Autodesk Inventor part; units mm, degrees
ref_plane "YZ Plane" through (0, 0, 0) normal (1, 0, 0) x (0, 1, 0)
ref_plane "XZ Plane" through (0, 0, 0) normal (0, 1, 0) x (-1, 0, 0)
ref_plane "XY Plane" through (0, 0, 0) normal (0, 0, 1) x (1, 0, 0)
sketch "Sketch3" plane through (0, 0, 0) normal (0, 1, 0) x (-1, 0, 0)
  line L0 (0, 0) -> (35, 0)
  line L1 (35, 0) -> (35, -45)
  line L2 (35, -45) -> (0, -45)
  line L3 (0, -45) -> (0, 0)
  circle A0 centre (25, -10.5) radius 8.5
  circle A1 centre (25, -34.5) radius 8.5
  line L4 (35, 0) -> (38, 0)
  line L5 (38, 0) -> (38, -45)
  line L6 (38, -45) -> (38, -48)
  line L7 (38, -48) -> (0, -48)
  line L8 (0, -48) -> (-3, -48)
  line L9 (-3, -48) -> (-3, 0)
  line L10 (-3, 0) -> (-3, 3)
  line L11 (-3, 3) -> (38, 3)
  line L12 (38, 3) -> (38, 0)
  dimension "d26" = 45
  dimension "d27" = 35
  dimension "d31" = 17
  dimension "d32" = 17
  dimension "d33" = 3
  dimension "d34" = 3
  dimension "d35" = 3
  dimension "d36" = 3
extrude "Extrusion3" add sketch "Sketch3" along normal blind 3 contours L0 L1 L2 L3
extrude "Extrusion4" add sketch "Sketch3" along normal blind 28 contours L5 L6 L7 L8 L9 L10 L11 L12
sketch "Sketch4" plane through (0, 28, 0) normal (0, 1, 0) x (1, 0, 0)
  line L0 (-38, 48) -> (-38, -3)
  line L1 (-38, -3) -> (2.7105, -3)
  line L2 (-38, -3) -> (3, -3)
  line L3 (3, 48) -> (-38, 48)
  line L4 (3, -3) -> (3, 48)
  line L5 (-38, 48) -> (3, 48)
  point P0 (0, 0)
  dimension "d41" = 51
  dimension "d43" = 41
properties part number "ultrasonido"
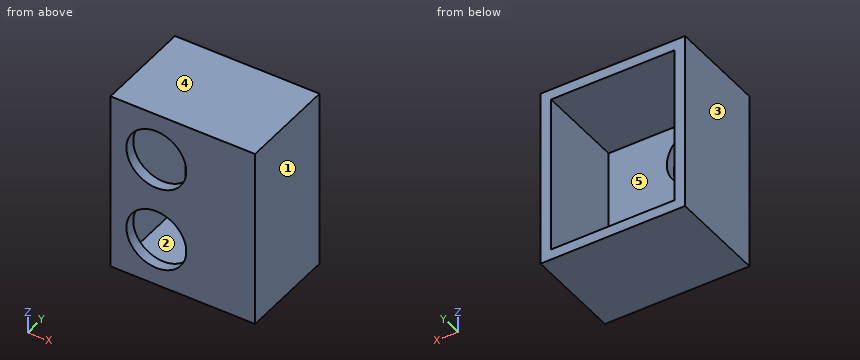
The model under review builds one solid part; all positions refer to its coordinate system, in mm. Face numbers are marked on the shaded views. A direction names the side the tool comes from. Coordinates: 2 decimals unless noted, no trailing zeros. Write each loop counter-clockwise with the first axis right and the second up, starting at its lowest first coordinate (ties: lowest second). Pieces come first, ordered by that corner, then holes. Notation, with made-up numbers: (27, -39.75) - (37, -39.75) arc R12 ccw to (37, -26.75) - close; hole circle Ø10 at (50.5, 11.25). An arc over 180 degrees is marked (long way). Answer as CSV lines item,"result".
(1) We need section A-A (y = 4.25). Give the boundary of the cut face in (x, z).
Data:
outline,"(-38, -48) - (3, -48) - (3, 3) - (-38, 3) - close; hole (-35, -45) - (0, -45) - (0, 0) - (-35, 0) - close"
(2) Mouldability with a two-part tool opening along Z and no side actions: class the marked faces 3, 4 and 5 as pulls with the +Z half, pulls with the -Z half, needs draft (parallel to the pull), parting line crosses it, or undercut.
Data:
face 3,"needs draft"
face 4,"pulls with the +Z half"
face 5,"undercut"
(3) For line 1 along Z through (x, y) = (-25, 1.3); line 2 along Z through (x, y) = (-33, 7); line 3 along X through (y, z) = (5.75, -44.5), list the stretches that pass through material, from the lowest coordinate up. Write a range as [from, to].
Data:
line 1,"z = [-48, -43], [-26, -19], [-2, 3]"
line 2,"z = [-48, -45], [0, 3]"
line 3,"x = [-38, -35], [0, 3]"
(4) We need section D-D (x = -9). Give the boundary of the cut face in (y, z).
Data:
outline,"(0, -48) - (28, -48) - (28, -45) - (3, -45) - (3, 0) - (28, 0) - (28, 3) - (0, 3) - close"
(5) We need section C-C (z = -22). Give the boundary of the cut face in (x, y), plus the area to 3 significant figures.
Data:
outline,"(-38, 0) - (3, 0) - (3, 28) - (0, 28) - (0, 3) - (-35, 3) - (-35, 28) - (-38, 28) - close"
area,"273 mm2"
(6) Clearance check with a flat-ended pin moving along its axis: pin 1 Ø19.5 at (x, z) = (-25, -10.5) entering from +Y. State where the tip first meets the part, or that it passes through.
Data:
pin 1,"stops at y = 3"
(7) Tool access review of the marked faces 1 and 2: name each direction out of +Z, -Z, +X, -X, +Y, -Y from which nothing blocks a thin tool from reaching the whole face with its end or side.
Data:
face 1,"+Z, -Z, +X, +Y, -Y"
face 2,"+Y"
(8) We need section B-B (z = -13). Give the boundary of the cut face in (x, y), plus the area to 3 significant figures.
Data:
outline,"(-38, 0) - (-33.12, 0) - (-33.12, 3) - (-35, 3) - (-35, 28) - (-38, 28) - close; (-16.88, 0) - (3, 0) - (3, 28) - (0, 28) - (0, 3) - (-16.88, 3) - close"
area,"224 mm2"
